Here's how the part is built. I have some questions about the finished solid (model axes, mm). Round coordinates to 2 decimals unless told otherwise and drop trailing zeros. Write each loop counter-clockwise with the first axis right and the second up, starting at its lowest first coordinate (ties: lowest second). Pieces come first, ordered by that corner, then holes. Notation, with made-up numbers: (6.5, 33.5) -> (47.5, 33.5) arc R24 ccw to (47.5, 67.5) -> close; hole circle Ø5 at (14, 46.25). An arc over 180 degrees is marked (long way). Answer as CSV lines item,"result".
from build123d import *

# Parameters (mm, degrees)
F3_DEPTH = 3
F4_DEPTH = 3
F5_DEPTH = 3.001


with BuildPart() as f3:
    # F0 (on Top) → F3 (new body)
    with BuildSketch(Plane.XY):
        with BuildLine():
            ThreePointArc((-233.3171, 564.475152), (-118.935157, 599.10224), (0, 610.7938))
            Line((0, 610.7938), (0, 814.4002))
            ThreePointArc((0, 814.4002), (-158.581858, 798.811292), (-311.092701, 752.64136))
            Line((-311.092701, 752.64136), (-233.3171, 564.475152))
        make_face()
        Polygon((-214.805697, 592.145084), (-208.825489, 594.280408), (-207.816675, 591.455112), (-213.796883, 589.319788), align=None, mode=Mode.SUBTRACT)
        Polygon((-155.117917, 607.408719), (-155.845492, 610.319154), (-149.685071, 611.859189), (-148.957495, 608.948754), align=None, mode=Mode.SUBTRACT)
        Polygon((-94.95078, 619.670291), (-95.390136, 622.637944), (-89.108603, 623.567915), (-88.669247, 620.600262), align=None, mode=Mode.SUBTRACT)
        Polygon((-33.872704, 625.986869), (-34.019626, 628.983269), (-27.677246, 629.294254), (-27.530324, 626.297854), align=None, mode=Mode.SUBTRACT)
    extrude(amount=F3_DEPTH)

    # F2 (on Top) → F4 (join)
    with BuildSketch(Plane.XY):
        Polygon((9, 785.9494), (9, 776.9494), (12, 776.9494), (12, 788.9494), (0, 788.9494), (0, 785.9494), align=None)
        Polygon((9, 735.0478), (9, 726.0478), (12, 726.0478), (12, 738.0478), (0, 738.0478), (0, 735.0478), align=None)
        Polygon((12, 636.2446), (0, 636.2446), (0, 633.2446), (9, 633.2446), (9, 624.2446), (12, 624.2446), align=None)
        Polygon((9, 684.1462), (9, 675.1462), (12, 675.1462), (12, 687.1462), (0, 687.1462), (0, 684.1462), align=None)
    extrude(amount=F4_DEPTH)

    # F2 (on Top) → F5 (cut, through all)
    with BuildSketch(Plane.XY):
        Polygon((-227.36518, 581.489807), (-231.94906, 592.579805), (-243.039057, 587.995925), (-241.893087, 585.223425), (-233.575589, 588.661335), (-230.137679, 580.343837), align=None)
        Polygon((-285.696882, 722.614463), (-290.280762, 733.70446), (-301.37076, 729.120581), (-300.22479, 726.348081), (-291.907292, 729.785991), (-288.469382, 721.468493), align=None)
        Polygon((-251.392961, 639.621356), (-262.482958, 635.037477), (-261.336988, 632.264977), (-253.01949, 635.702887), (-249.58158, 627.385389), (-246.809081, 628.531359), align=None)
        Polygon((-280.780889, 679.306529), (-272.463391, 682.744439), (-269.025481, 674.426941), (-266.252982, 675.572911), (-270.836861, 686.662908), (-281.926859, 682.079029), align=None)
    extrude(amount=F5_DEPTH, mode=Mode.SUBTRACT)


solid = f3.part
Item 1: Will these pins go through, and if not, where does the flat tip stop? pin 1 (1.5 mm diameter, centred on y = 731.5, z = 1.5, fed in from -X); pin 2 (1 mm diameter, centred on x = -63.5, y = 605, fed in from -Z); pin 3 (0.9 mm diameter, centred on y = 621, z = 2, fed in from +X); pin 4 (1.5 mm diameter, centred on y = 722.5, z = 1, fed in from -X).
Results found:
pin 1,"stops at x = -302.66"
pin 2,"passes through"
pin 3,"stops at x = 0"
pin 4,"stops at x = -298.94"
Item 2: If we mould it in two halves opening along Z, with no side actions, what happens to faces 1 (the flat face through (-116, 691, 0)), 2 (the flat face through (-116, 691, 3)), 3 (the flat face through (-271.76, 657.48, 1.48))? For each: pulls with the +Z half, pulls with the -Z half, needs draft (parallel to the pull), parting line crosses it, or undercut.
Results found:
face 1,"pulls with the -Z half"
face 2,"pulls with the +Z half"
face 3,"needs draft"
Item 3: Suppose I cut it at A-A, the plane y = 782. List the corners of the cut face in (x, z) for me.
Results found:
outline,"(-227.43, 0) -> (0, 0) -> (0, 3) -> (-227.43, 3) -> close; (9, 0) -> (12, 0) -> (12, 3) -> (9, 3) -> close"
Item 4: Suppose I cut it at B-B, the plane z = 1.85. State how many separate pieces and enclosed holes the cut face has, then the cut area to 3 significant figures.
Results found:
separate pieces,"1"
enclosed holes,"4"
area,"56,800 mm²"
Item 5: I need wall thicknesses on L1, parallel to X at y = 630, z = 1.6; L2, parallel to X at y = 723, z = 2.4; L3, parallel to X at y = 622, z = 1.55. Which ranges of each line are inside material? Lowest first, please.
Results found:
L1,"x = -260.4 to -250.66, -247.42 to 0, 9 to 12"
L2,"x = -298.84 to -289.1, -285.86 to 0"
L3,"x = -257.09 to -95.3, -88.88 to 0"
Item 6: Suppose I cut it at C-C, the plane x = -68.5. List the corners of the cut face in (y, z) for me, then the cut area to 3 significant figures.
Results found:
outline,"(606.94, 0) -> (811.51, 0) -> (811.51, 3) -> (606.94, 3) -> close"
area,"614 mm²"
Item 7: Suppose I cut it at D-D, the plane y = 665. List the corners of the cut face in (x, z) for me.
Results found:
outline,"(-274.87, 0) -> (0, 0) -> (0, 3) -> (-274.87, 3) -> close"
